Geometry: see drawing. Coordinates: mm, zero at the bounding-box minimum. A direction names the side the tool comes from. Give positions to 0.01 mm unless a question says otherwise; leave off trailing zeros. Order: outer loops, then holes, each group sorted by start corner. A loop starts at its lowest first (then second) coordinate and runs counter-clockwise, first axis right, second up. Notation, with made-up numbers: (13.25, 8.5) - (20.25, 8.5) arc R27 cw to (20.25, 43.5) - close; hole circle Ø2 at (40, -32). An arc over 180 degrees is marked (long way). One line per item, written item: value.
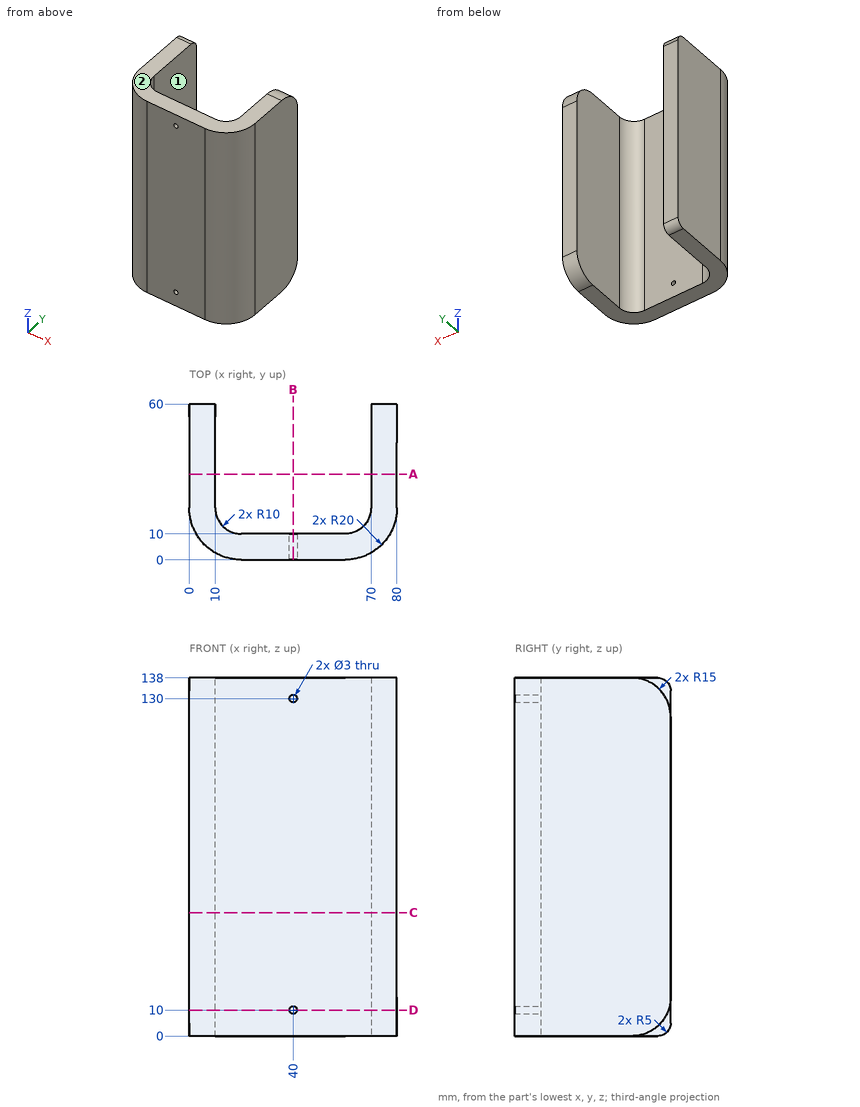
1) Section D-D, the plane z = 10. Return loops of the section in (x, y).
Answers below:
outline: (0, 20) arc R20 ccw to (20, 0) - (38.5, 0) - (38.5, 10) - (20, 10) arc R10 cw to (10, 20) - (10, 60) - (0, 60) - close; (41.5, 0) - (60, 0) arc R20 ccw to (80, 20) - (80, 59.14) - (70, 59.14) - (70, 20) arc R10 cw to (60, 10) - (41.5, 10) - close
2) Section A-A, the plane y = 33. Return loops of the section in (x, z), then the cut area to 3 significant figures.
Answers below:
outline: (0, 0) - (10, 0) - (10, 138) - (0, 138) - close; (70, 0) - (80, 0) - (80, 138) - (70, 138) - close
area: 2,760 mm^2
3) Material intervals for line 1 along Z through (x, y) = (40, 5); line 2 along X through (y, z) = (40.5, 37); line 3 along Y through (x, z) = (23.5, 72.5), sorted ascending.
Answers below:
line 1: 0 to 8.5, 11.5 to 128.5, 131.5 to 138
line 2: 0 to 10, 70 to 80
line 3: 0 to 10
4) Set-up query: the marked faces 1 and 2. Return all of +Z, -Z, +X, -X, +Y, -Y with unobstructed straight access to the full face (end or side cutting, diameter ignored); none if empty.
Answers below:
face 1: +Z, -Z, +Y
face 2: +Z, +X, -X, +Y, -Y
5) Section B-B, the plane x = 40. Return loops of the section in (y, z).
Answers below:
outline: (0, 0) - (10, 0) - (10, 8.5) - (0, 8.5) - close; (0, 11.5) - (10, 11.5) - (10, 128.5) - (0, 128.5) - close; (0, 131.5) - (10, 131.5) - (10, 138) - (0, 138) - close
6) First-contact query: pin 1 (1 mm diameter, centred on x = 15.5, z = 56.5, fed in from -Y); pin 2 (6 mm diameter, centred on x = 15.5, y = 21, fed in from +Z); pin 3 (12 mm diameter, centred on y = 9, z = 27, fed in from +X). Flat tips, straight axial feed; report the tip coordinate or a pass-through.
Answers below:
pin 1: y = 0.4
pin 2: through
pin 3: x = 79.36
7) Section C-C, the plane z = 47.5. Return loops of the section in (x, y), then the cut area to 3 significant figures.
Answers below:
outline: (0, 20) arc R20 ccw to (20, 0) - (60, 0) arc R20 ccw to (80, 20) - (80, 60) - (70, 60) - (70, 20) arc R10 cw to (60, 10) - (20, 10) arc R10 cw to (10, 20) - (10, 60) - (0, 60) - close
area: 1,670 mm^2
